The listing builds one solid part. Answer for the finished solid, in the listing's coordinates (mm). A direction names the side the tool comes from. Round coordinates to 2 decimals unless told otherwise and drop trailing zeros. Order: outer loops, then holes, each group sorted by start corner. A loop starts at its lowest first (then second) coordinate and runs counter-clockwise, first axis right, second up. Notation, with made-up numbers: (-17, -13.5) -> (24, -13.5) arc R20 cw to (24, 14.5) -> close; hole circle Ø2 at (51.5, 60). An arc over 180 degrees is marked (long way). Answer in a Markdown table with one row per item. Add a question column.
```python
from build123d import *

# Parameters (mm, degrees)
CROQUIS1_R              = 1.55
SALIENTE_EXTRUIR1_DEPTH = 15
REDONDEO1_R             = 2
CROQUIS10_R             = 1.5
CORTAR_EXTRUIR1_DEPTH   = 56.90169959


with BuildPart() as part:
    # Croquis1 → Saliente-Extruir1 (new body)
    with BuildSketch(Plane.XY):
        Polygon((-5, 25), (-10, 30), (-10, 50), (10, 50), (10, 30), (5, 25), (5, -5), (-5, -5), align=None)
        Circle(CROQUIS1_R, mode=Mode.SUBTRACT)
    extrude(amount=SALIENTE_EXTRUIR1_DEPTH)

    # Croquis8 → Cortar-Recubrir1 section 0
    with BuildSketch(Plane.XY.offset(15)):
        with BuildLine():
            Line((5, 50), (-5, 50))
            Line((-5, 50), (-5, 35))
            Line((-5, 35), (5, 35))
            Line((5, 35), (5, 50))
        make_face()
    # Croquis9 → Cortar-Recubrir1 section 1
    with BuildSketch(Plane(origin=(0, 0, 0), x_dir=(-1, 0, 0), z_dir=(0, 0, -1))):
        with BuildLine():
            Line((5, 50), (-5, 50))
            Line((-5, 50), (-5, 40))
            Line((-5, 40), (5, 40))
            Line((5, 40), (5, 50))
        make_face()
    loft(mode=Mode.SUBTRACT)

    # Redondeo1
    redondeo1_edges = [part.edges().sort_by_distance(p)[0] for p in [
        (0, -5, 0),
        (5, 25, 7.5),
        (-5, 25, 7.5),
        (-10, 30, 7.5),
        (10, 30, 7.5),
        (0, -5, 15),
    ]]
    fillet(redondeo1_edges, radius=REDONDEO1_R)

    # Croquis10 → Cortar-Extruir1 (cut, through all)
    with BuildSketch(Plane(origin=(10, 0, 0), x_dir=(0, 0, -1), z_dir=(1, 0, 0))):
        with Locations(Location((-7.5, 45, 0), (0, 0, 90))):
            Circle(CROQUIS10_R)
        with BuildLine():
            Line((-10, -5), (-10, 4.5))
            ThreePointArc((-10, 4.5), (-7.5, 7), (-5, 4.5))
            Line((-5, 4.5), (-5, -5))
            ThreePointArc((-5, -5), (-7.5, -7.5), (-10, -5))
        make_face()
        with BuildLine():
            Line((-17.5, 9.5), (-15, 9.5))
            ThreePointArc((-15, 9.5), (-13.629356685, 26), (-15, 42.5))
            ThreePointArc((-15, 42.5), (-7.5, 50), (0, 42.5))
            ThreePointArc((0, 42.5), (-1.370643315, 26), (0, 9.5))
            Line((0, 9.5), (2.5, 9.5))
            Line((2.5, 9.5), (2.5, 51.5))
            Line((2.5, 51.5), (-17.5, 51.5))
            Line((-17.5, 51.5), (-17.5, 9.5))
        make_face()
    extrude(amount=-CORTAR_EXTRUIR1_DEPTH, mode=Mode.SUBTRACT)


solid = part.part
```
Item 1: A tool of negligible diameter and unlimited length cuts with its end or side. For faces 1 (the face through (5.15, 24.93, 7.59)), 2 (the face through (-5, 9, 7)), 3 (the face through (1.18, -1.24, 5)), from which of +Z, -Z, +X, -X, +Y, -Y can it reach the whole face along a straight path? Write none if from no direction.
Item 2: For a pull along Y with two mould halves and no side action, classify faces 4 (the face through (-7.46, 50, 7.66)), 5 (the face through (-10, 40, 7)), 6 (the face through (0.14, 25.77, 13.63)) as released by +Y, released by -Y, zero draft, split by the parting line, or undercut.
Item 3: Find the intervals of material crossed by probe 1 along X at (y, z) = (0, 2); probe 2 along Z at (x, y) = (6.5, 45); probe 3 along Y at (x, z) = (7.9, 7.5), in increasing order. Write a range as [from, to].
Item 4: The part is cut by section B-B, the plane x = -4.5. Give the vertices of the cut face in (y, z).
Item 5: Flat-ended cylindrical pins translate along their axes: P1, Ø5, axis at y = 8.5, z = 3.5, coming from the +X side; P2, Ø2.5, axis at x = 0, y = 0, coming from the -Z side. Find the tip coordinate at first contact, or state that the pin passes through.
Item 6: The part is cut by section A-A, the plane y = 0. Give the vertices of the cut face in (x, z), and give its area (3 significant figures).
Item 7: The part is cut by section C-C, the plane z = 7.5. State how many separate pieces and enclosed holes the cut face has, and give its area (3 significant figures).
Item 8: The part is cut by section D-D, the plane x = 6.75. Give the vertices of the cut face in (y, z), and give its area (3 significant figures).
Resolved:
| question | item | result |
|---|---|---|
| 1 | face 1 | +Z, -Z, +X, -Y |
| 1 | face 2 | +Z, -Z, -X, -Y |
| 1 | face 3 | +X, -X, -Y |
| 2 | face 4 | released by +Y |
| 2 | face 5 | zero draft |
| 2 | face 6 | undercut |
| 3 | probe 1 | [-5, -1.55], [1.55, 5] |
| 3 | probe 2 | [0.43, 6], [9, 14.57] |
| 3 | probe 3 | [27.9, 43.5], [46.5, 50] |
| 4 | outline | (-5, 2) arc R2 ccw to (-3, 0) -> (9.5, 0) arc R100 cw to (39.87, 0.4) -> (35.31, 14.06) arc R100 cw to (9.5, 15) -> (-3, 15) arc R2 ccw to (-5, 13) -> (-5, 10) -> (4.5, 10) arc R2.5 cw to (4.5, 5) -> (-5, 5) -> close |
| 5 | P1 | x = 5 |
| 5 | P2 | through |
| 6 | outline | (-5, 0) -> (-1.55, 0) -> (-1.55, 5) -> (-5, 5) -> close; (-5, 10) -> (-1.55, 10) -> (-1.55, 15) -> (-5, 15) -> close; (1.55, 0) -> (5, 0) -> (5, 5) -> (1.55, 5) -> close; (1.55, 10) -> (5, 10) -> (5, 15) -> (1.55, 15) -> close |
| 6 | area | 69.0 mm2 |
| 7 | separate pieces | 3 |
| 7 | enclosed holes | 0 |
| 7 | area | 500 mm2 |
| 8 | outline | (26.75, 1.37) arc R100 cw to (42.5, 0) arc R7.5 ccw to (42.5, 15) arc R100 cw to (26.75, 13.63) -> close; hole circle Ø3 at (45, 7.5) |
| 8 | area | 289 mm2 |
